from build123d import *

# Parameters (mm, degrees)
F1_DEPTH = 25.4
F2_W     = 110.45
F2_H     = 19.5
F3_DEPTH = 19
F4_R     = 15


with BuildPart() as f1:
    # F0 (on Top) → F1 (new body)
    with BuildSketch(Plane.XY):
        with BuildLine():
            Line((0, 50), (0, 0))
            Line((0, 0), (115, 0))
            Line((115, 0), (115, 21))
            Line((115, 21), (36.155032, 57.766013))
            ThreePointArc((36.155032, 57.766013), (16.773652, 59.953206), (0, 50))
        make_face()
    extrude(amount=F1_DEPTH)

    # F2 (on face) → F3 (cut)
    with BuildSketch(Plane.XZ):
        with Locations((59.775, 13.15)):
            Rectangle(F2_W, F2_H)
    extrude(amount=-F3_DEPTH, mode=Mode.SUBTRACT)

    # F4
    f4_edges = [f1.edges().sort_by_distance(p)[0] for p in [
        (4.55, 19, 13.15),
    ]]
    fillet(f4_edges, radius=F4_R)


solid = f1.part
Model file for the job. Use its own axes, mm. A direction names the side the tool comes from. Round coordinates to 2 decimals unless told otherwise and drop trailing zeros. Order: outer loops, then holes, each group sorted by start corner. A loop starts at its lowest first (then second) coordinate and runs counter-clockwise, first axis right, second up.
(1) Band-saw the part on B-B (x = 23.5). List the corners of the cut face in (y, z) (3 decimals), then the cut area to 3 significant figures.
(2) Pin check, flat tips, straight feed: pin 1 (6 mm diameter, centred on y = 40, z = 9, fed in from -X); pin 2 (4.5 mm diameter, centred on y = 1.5, z = 16, fed in from +X); pin 3 (2 mm diameter, centred on x = 51.5, z = 22, fed in from +Y); pin 4 (10 mm diameter, centred on x = 83.5, z = 15.5, fed in from -Y). Stop position of each tip, or through.
(3) Band-saw the part on A-A (z = 7.25). List the corners of the cut face in (x, y).
(4) Band-saw the part on D-D (z = 2.25). List the corners of the cut face in (x, y), then the cut area to 3 significant figures.
(5) Band-saw the part on C-C (y = 33). List the corners of the cut face in (x, z), then the cut area to 3 significant figures.
(6) Pull direction Z, two halves, no side cores. Call faces 1 (the face through (8.83, 14.49, 13.29)), 2 (the face through (67, 19, 13)), 3 (the face through (53, 0, 3)), 4 (the face through (44, 24, 0)): released by +Z, released by -Z, zero draft, split by the parting line, or undercut.
(7) 3-axis set-ups, long thin cutter, end or side, ignore diameter. For faces 5 (the face through (115, 20, 13)), 6 (the face through (4.55, 2, 13)): which of +Z, -Z, +X, -X, +Y, -Y reach the whole face in a straight line?
(8) Drill centre lines: line 1 (Z direction, x = 27, y = 14.5); line 2 (Y direction, x = 98.5, z = 21); line 3 (Y direction, x = 50, z = 4.5). Where is each one in solid material? Low to high.
Verdict:
1. outline: (0, 0) - (60.635, 0) - (60.635, 25.4) - (0, 25.4) - (0, 22.9) - (19, 22.9) - (19, 3.4) - (0, 3.4) - close
1. area: 1,170 mm2
2. pin 1: stops at x = 0
2. pin 2: stops at x = 4.55
2. pin 3: stops at y = 51.08
2. pin 4: stops at y = 19
3. outline: (0, 0) - (4.55, 0) - (4.55, 4) arc R15 cw to (19.55, 19) - (115, 19) - (115, 21) - (36.16, 57.77) arc R30.64 ccw to (0, 50) - close
4. outline: (0, 0) - (115, 0) - (115, 21) - (36.16, 57.77) arc R30.64 ccw to (0, 50) - close
4. area: 5,210 mm2
5. outline: (0, 0) - (89.27, 0) - (89.27, 25.4) - (0, 25.4) - close
5. area: 2,270 mm2
6. face 1: undercut
6. face 2: undercut
6. face 3: zero draft
6. face 4: released by -Z
7. face 5: +Z, -Z, +X, +Y, -Y
7. face 6: +X, -Y
8. line 1: z = 0 to 3.4, 22.9 to 25.4
8. line 2: y = 19 to 28.69
8. line 3: y = 19 to 51.31
